CAD build for the part. Positions are in the model's coordinates, mm. Round coordinates to 2 decimals unless told otherwise and drop trailing zeros. Loops run counter-clockwise (first coordinate to the right, second up) from the corner with the lowest first, then second, coordinate; pieces in that order, holes last. Notation, with made-up numbers: (87, 65) - (112, 65) arc R16 cw to (112, 74) - close; hole circle Ø1 at (-2, 52.25). An arc over 180 degrees is marked (long way). One line per question, with ' | ' between items.
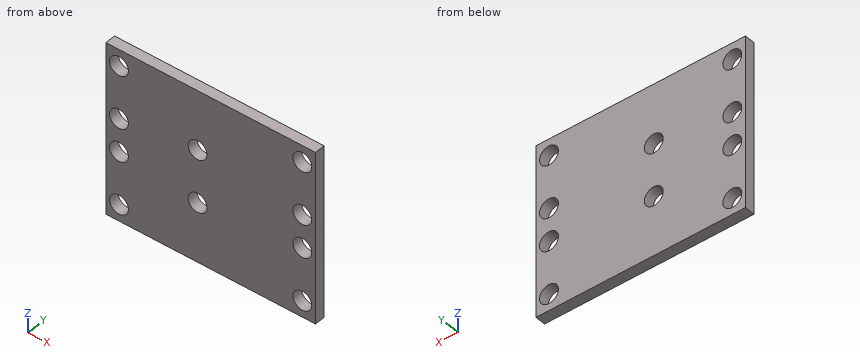
```python
from build123d import *

# Parameters (mm, degrees)
SKETCH1_R           = 2.286
BOSS_EXTRUDE1_DEPTH = 2.54


with BuildPart() as part:
    # Sketch1 → Boss-Extrude1 (new body)
    with BuildSketch(Plane(origin=(0, 0, 0), x_dir=(1, 0, 0), z_dir=(0, 1, 0))):
        Polygon((-25.4, -14.2875), (-25.4, -26.9875), (25.4, -26.9875), (25.4, -14.2875), (25.4, 14.2875), (-25.4, 14.2875), align=None)
        with Locations(Location((-22.225, 10.31875, 0), (0, 0, 270))):
            Circle(SKETCH1_R, mode=Mode.SUBTRACT)
        with Locations(Location((-22.225, -10.31875, 0), (0, 0, 270))):
            Circle(SKETCH1_R, mode=Mode.SUBTRACT)
        with Locations(Location((22.225, -10.31875, 0), (0, 0, 270))):
            Circle(SKETCH1_R, mode=Mode.SUBTRACT)
        with Locations(Location((22.225, 10.31875, 0), (0, 0, 270))):
            Circle(SKETCH1_R, mode=Mode.SUBTRACT)
        with Locations(Location((-22.225, -2.38125, 0), (0, 0, 270))):
            Circle(SKETCH1_R, mode=Mode.SUBTRACT)
        with Locations(Location((-22.225, -23.01875, 0), (0, 0, 270))):
            Circle(SKETCH1_R, mode=Mode.SUBTRACT)
        with Locations(Location((22.225, -23.01875, 0), (0, 0, 270))):
            Circle(SKETCH1_R, mode=Mode.SUBTRACT)
        with Locations(Location((22.225, -2.38125, 0), (0, 0, 270))):
            Circle(SKETCH1_R, mode=Mode.SUBTRACT)
        with Locations(Location((-3.175, 0, 0), (0, 0, 270))):
            Circle(SKETCH1_R, mode=Mode.SUBTRACT)
        with Locations(Location((-3.175, -12.7, 0), (0, 0, 270))):
            Circle(SKETCH1_R, mode=Mode.SUBTRACT)
    extrude(amount=BOSS_EXTRUDE1_DEPTH)


solid = part.part
```
(1) Probe L1, parallel to Z at x = 23.5, y = 0.5; L2, parallel to Z at x = -3.5, y = 2.05; L3, parallel to X at y = 1.95, z = 21. List the from-to ranges inside material, lowest first.
Results found:
L1: z = -14.29 to -12.22, -8.42 to 0.48, 4.28 to 8.42, 12.22 to 21.12, 24.92 to 26.99 | L2: z = -14.29 to -2.26, 2.26 to 10.44, 14.96 to 26.99 | L3: x = -25.4 to -23.3, -21.15 to 21.15, 23.3 to 25.4
(2) Cut at A-A, the plane y = 1.4. State how many separate pieces and enclosed holes the cut face has, then the cut area to 3 significant figures.
Results found:
separate pieces: 1 | enclosed holes: 10 | area: 1,930 mm²
(3) Cut at B-B, the plane z = -11. Write the cut outline in (x, y).
Results found:
outline: (-25.4, 0) - (-24.41, 0) - (-24.41, 2.54) - (-25.4, 2.54) - close; (-20.04, 0) - (20.04, 0) - (20.04, 2.54) - (-20.04, 2.54) - close; (24.41, 0) - (25.4, 0) - (25.4, 2.54) - (24.41, 2.54) - close
(4) Drop a flat-ended pin along its axis: P1, Ø7.5, axis at x = -3.175, z = 12.7, coming from the -Y side. Give the stop position or say it passes through.
Results found:
P1: stops at y = 0
